Model file for the job. Use its own axes, mm. Coordinates: 2 decimals unless noted, no trailing zeros. Loops run counter-clockwise (first coordinate to the right, second up) from the corner with the lowest first, then second, coordinate; pieces in that order, holes last.
from build123d import *

# Parameters (mm, degrees)
MODEL_R                 = 1.5
SALIENTE_EXTRUIR1_DEPTH = 3


with BuildPart() as part:
    # Model → Saliente-Extruir1 (new body)
    with BuildSketch(Plane.XY):
        with BuildLine():
            Line((-105.943383637, 101.056539338), (-105.943383637, 74.056539338))
            ThreePointArc((-105.943383637, 74.056539338), (-104.625364152, 70.874558823), (-101.443383637, 69.556539338))
            Line((-101.443383637, 69.556539338), (-74.443383637, 69.556539338))
            ThreePointArc((-74.443383637, 69.556539338), (-72.721308191, 69.899081442), (-71.261403122, 70.874558823))
            Line((-71.261403122, 70.874558823), (-104.625364152, 104.238519853))
            ThreePointArc((-104.625364152, 104.238519853), (-105.600841533, 102.778614784), (-105.943383637, 101.056539338))
        make_face()
        with Locations((-101.443383637, 92.056539338)):
            Circle(MODEL_R, mode=Mode.SUBTRACT)
        with Locations((-101.443383637, 83.056539338)):
            Circle(MODEL_R, mode=Mode.SUBTRACT)
        with Locations((-92.443383637, 83.056539338)):
            Circle(MODEL_R, mode=Mode.SUBTRACT)
        with Locations((-101.443383637, 74.056539338)):
            Circle(MODEL_R, mode=Mode.SUBTRACT)
        with Locations((-92.443383637, 74.056539338)):
            Circle(MODEL_R, mode=Mode.SUBTRACT)
        with Locations((-83.443383637, 74.056539338)):
            Circle(MODEL_R, mode=Mode.SUBTRACT)
    extrude(amount=SALIENTE_EXTRUIR1_DEPTH)


solid = part.part
Q1. Slice it at C-C (y = 92.5). List the corners of the cut face in (x, z), and give its area (3 significant figures).
Answers:
outline: (-105.94, 0) - (-102.88, 0) - (-102.88, 3) - (-105.94, 3) - close; (-100.01, 0) - (-92.89, 0) - (-92.89, 3) - (-100.01, 3) - close
area: 30.6 mm2
Q2. Drill centre lines: line 1 (X direction, y = 73.5, z = 2.3); line 2 (X direction, y = 75, z = 1.1); line 3 (Y direction, x = -101, z = 2). Where is each one in solid material? Low to high.
Answers:
line 1: x = -105.91 to -102.84, -100.05 to -93.84, -91.05 to -84.84, -82.05 to -73.89
line 2: x = -105.94 to -102.61, -100.28 to -93.61, -91.28 to -84.61, -82.28 to -75.39
line 3: y = 69.56 to 72.62, 75.49 to 81.62, 84.49 to 90.62, 93.49 to 100.61
Q3. Mould opens along X. For faces 1 (the flat face through (-93, 79, 3)), 2 (the cylindrical face through (-91.06, 82.48, 1.48)), 3 (the cylindrical face through (-104.66, 70.91, 1.48)) say: +X half, -X half, draft (parallel to the pull), parting line (faces both ways), or undercut.
Answers:
face 1: draft
face 2: undercut
face 3: -X half
Q4. Slice it at A-A (y = 74.5). List the corners of the cut face in (x, z), and give its area (3 significant figures).
Answers:
outline: (-105.94, 0) - (-102.88, 0) - (-102.88, 3) - (-105.94, 3) - close; (-100.01, 0) - (-93.88, 0) - (-93.88, 3) - (-100.01, 3) - close; (-91.01, 0) - (-84.88, 0) - (-84.88, 3) - (-91.01, 3) - close; (-82.01, 0) - (-74.89, 0) - (-74.89, 3) - (-82.01, 3) - close
area: 67.4 mm2
Q5. Slice it at B-B (z = 2). List the corners of the cut face in (x, y), and give its area (3 significant figures).
Answers:
outline: (-105.94, 74.06) arc R4.5 ccw to (-101.44, 69.56) - (-74.44, 69.56) arc R4.5 ccw to (-71.26, 70.87) - (-104.63, 104.24) arc R4.5 ccw to (-105.94, 101.06) - close; hole circle Ø3 at (-101.44, 74.06); hole circle Ø3 at (-101.44, 83.06); hole circle Ø3 at (-101.44, 92.06); hole circle Ø3 at (-92.44, 74.06); hole circle Ø3 at (-92.44, 83.06); hole circle Ø3 at (-83.44, 74.06)
area: 597 mm2
Q6. Slice it at D-D (x = -76.5). List the corners of the cut face in (y, z), and give its area (3 significant figures).
Answers:
outline: (69.56, 0) - (76.11, 0) - (76.11, 3) - (69.56, 3) - close
area: 19.7 mm2
Q7. Flat gauge pin, fed straight in: P1, Ø2.5, axis at x = -101.44, y = 74.06, coming from the +Z side. Where does the tip first touch, or does it go through?
Answers:
P1: passes through
